Could you check a few things on this model? Use its own coordinates, in mm. Give positions to 0.01 mm unless a question says otherwise; leave off trailing zeros. Write each loop counter-clockwise with the first axis right and the second up, starting at its lowest first coordinate (ties: lowest second). Pieces come first, ordered by that corner, then holes. Notation, with made-up numbers: M -32.75,16 L -9.75,16 A12 cw -9.75,21 Z; hole C 1,68 d9. An arc over 180 degrees is marked long. Use one line per item in the form item = value.
from build123d import *

# Parameters (mm, degrees)
SKETCH1_W           = 150
SKETCH1_H           = 150
BOSS_EXTRUDE1_DEPTH = 59
SKETCH2_W           = 111.9
SKETCH2_H           = 111.9
CUT_EXTRUDE1_DEPTH  = 60
SKETCH9_R           = 1.4
CUT_EXTRUDE4_DEPTH  = 20
CIRPATTERN1_COUNT   = 3
CIRPATTERN1_ANGLE   = 180
SKETCH10_W          = 111.9
SKETCH10_H          = 105.448295943
CUT_EXTRUDE6_DEPTH  = 60
SKETCH12_W          = 150
SKETCH12_H          = 130.95
CUT_EXTRUDE7_DEPTH  = 60


with BuildPart() as part:
    # Sketch1 → Boss-Extrude1 (new body)
    with BuildSketch(Plane(origin=(0, 0, 0), x_dir=(1, 0, 0), z_dir=(0, 1, 0))):
        Rectangle(SKETCH1_W, SKETCH1_H)
    extrude(amount=-BOSS_EXTRUDE1_DEPTH)

    # Sketch2 → Cut-Extrude1 (cut, through all)
    with BuildSketch(Plane(origin=(0, 0, 0), x_dir=(1, 0, 0), z_dir=(0, 1, 0))):
        Rectangle(SKETCH2_W, SKETCH2_H)
    extrude(amount=-CUT_EXTRUDE1_DEPTH, mode=Mode.SUBTRACT)

    # Sketch9 → Cut-Extrude4 (cut)
    with BuildSketch(Plane.ZY.offset(75)):
        with Locations((-6.1, -7.25)):
            Circle(SKETCH9_R)
        with Locations((6.1, -7.25)):
            Circle(SKETCH9_R)
        with Locations((6.1, -15.25)):
            Circle(SKETCH9_R)
        with Locations((-6.1, -15.25)):
            Circle(SKETCH9_R)
    cut_extrude4 = extrude(amount=-CUT_EXTRUDE4_DEPTH, mode=Mode.SUBTRACT)

    # CirPattern1: Cut-Extrude4 ×3 about axis
    cirpattern1_axis = Axis((0, 0, 0), (0, 1, 0))
    for i in range(1, CIRPATTERN1_COUNT):
        add(cut_extrude4.rotate(cirpattern1_axis, i * CIRPATTERN1_ANGLE / (CIRPATTERN1_COUNT - 1)), mode=Mode.SUBTRACT)

    # Sketch10 → Cut-Extrude6 (cut, through all)
    with BuildSketch(Plane(origin=(0, 0, 0), x_dir=(1, 0, 0), z_dir=(0, 1, 0))):
        with Locations((0, 108.674147972)):
            Rectangle(SKETCH10_W, SKETCH10_H)
    extrude(amount=-CUT_EXTRUDE6_DEPTH, mode=Mode.SUBTRACT)

    # Sketch12 → Cut-Extrude7 (cut, through all)
    with BuildSketch(Plane(origin=(0, 0, 0), x_dir=(1, 0, 0), z_dir=(0, 1, 0))):
        with Locations((0, 9.525)):
            Rectangle(SKETCH12_W, SKETCH12_H)
    extrude(amount=-CUT_EXTRUDE7_DEPTH, mode=Mode.SUBTRACT)


solid = part.part
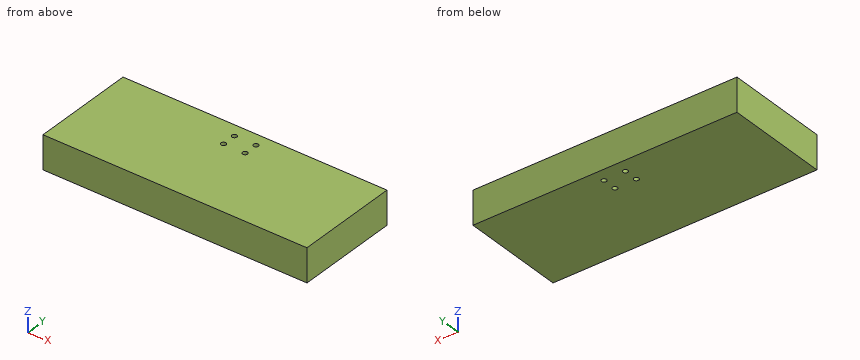
1) For pin 1 Ø2 at (x, y) = (-6.1, -15.25) entering from +Z, with a flat end and sliding along its axis, tell me the tip position at first contact or that it passes through.
Checked values:
pin_1 = through
2) I want a section at B-B, the plane y = -7.25. Please give me the cut outline in (x, z).
Checked values:
outline = M -75,55.95 L -7.5,55.95 L -7.5,75 L -75,75 Z; M -4.7,55.95 L 4.7,55.95 L 4.7,75 L -4.7,75 Z; M 7.5,55.95 L 75,55.95 L 75,75 L 7.5,75 Z
3) I want a section at A-A, the plane x = 6.1. Please give me the cut outline in (y, z), plus the area to 3 significant figures.
Checked values:
outline = M -59,55.95 L -16.65,55.95 L -16.65,75 L -59,75 Z; M -13.85,55.95 L -8.65,55.95 L -8.65,75 L -13.85,75 Z; M -5.85,55.95 L 0,55.95 L 0,75 L -5.85,75 Z
area = 1,020 mm2
4) If I drill on L1, parallel to Y at x = -6.1, z = 71; L2, parallel to X at y = -6, z = 71.25; L3, parallel to Y at x = 5.5, z = 71.75, over which ranges is the centre line in solid material (lowest first)?
Checked values:
L1 = -59 to -16.65, -13.85 to -8.65, -5.85 to 0
L2 = -75 to -6.73, -5.47 to 5.47, 6.73 to 75
L3 = -59 to -16.51, -13.99 to -8.51, -5.99 to 0
